Read the model definition and answer for the solid it produces. Units are mm, in the model's axes. Face numbers are marked on the shaded views. Give positions to 0.01 mm unless a question says otherwise; leave off trailing zeros. Order: outer loops, then holes, each group sorted by start corner. A loop starts at its lowest first (then second) coordinate and runs counter-clockwise, first axis right, second up.
```python
from build123d import *

# Parameters (mm, degrees)
F0_W     = 39
F0_H     = 55
F1_DEPTH = 25
F3_DEPTH = 25
F4_R     = 5


with BuildPart() as f1:
    # F0 (on Front) → F1 (new body)
    with BuildSketch(Plane.XZ):
        Rectangle(F0_W, F0_H)
    extrude(amount=F1_DEPTH)

    # F2 (on face) → F3 (cut)
    with BuildSketch(Plane.XZ.offset(25)):
        with BuildLine():
            Line((18.6, 27.5), (-18.6, 27.5))
            ThreePointArc((-18.6, 27.5), (-13.089826, 1.090185), (0, -22.5))
            ThreePointArc((0, -22.5), (13.089826, 1.090185), (18.6, 27.5))
        make_face()
    extrude(amount=-F3_DEPTH, mode=Mode.SUBTRACT)

    # F4
    f4_edges = [f1.edges().sort_by_distance(p)[0] for p in [
        (-19.5, -12.5, -27.5),
        (19.5, -12.5, -27.5),
    ]]
    fillet(f4_edges, radius=F4_R)


solid = f1.part
```
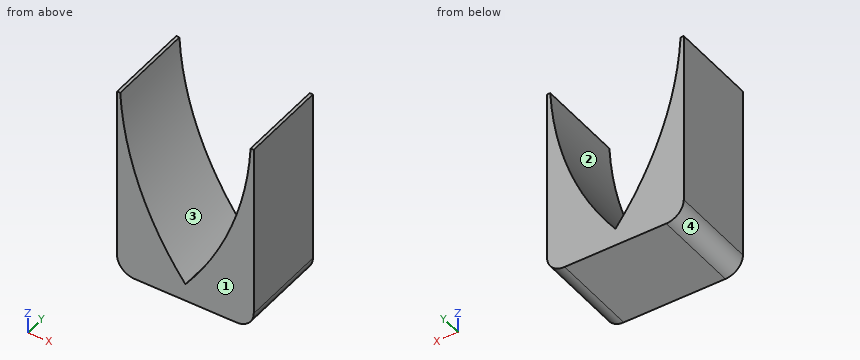
1) The part is cut by section B-B on y = -7.25. Determine the outline of the cut face in (x, z), and give its area (3 significant figures).
Final values:
outline: (-19.5, -22.5) arc R5 ccw to (-14.5, -27.5) - (14.5, -27.5) arc R5 ccw to (19.5, -22.5) - (19.5, 27.5) - (18.6, 27.5) arc R90 cw to (0, -22.5) arc R90 cw to (-18.6, 27.5) - (-19.5, 27.5) - close
area: 915 mm2
2) Consider L1, parallel to X at y = -4.75, z = 20; L2, parallel to X at y = -3.5, z = -10.5; L3, parallel to Z at x = 5, y = -14.5. Determine where each line is inside the solid, lowest interval first.
Final values:
L1: x = -19.5 to -17.87, 17.87 to 19.5
L2: x = -19.5 to -7.82, 7.82 to 19.5
L3: z = -27.5 to -15.32
3) The part is cut by section D-D on x = -12. Determine the outline of the cut face in (y, z).
Final values:
outline: (-25, -27.5) - (0, -27.5) - (0, -1.7) - (-25, -1.7) - close
4) For a pull along X with two mould halves and no side action, classify the marked faces 1, 2, 3 and 4 as released by +X, released by -X, zero draft, split by the parting line, or undercut.
Final values:
face 1: zero draft
face 2: undercut
face 3: undercut
face 4: released by -X
5) The part is cut by section C-C on z = -0.5. Determine the outline of the cut face in (x, y).
Final values:
outline: (-19.5, -25) - (-12.48, -25) - (-12.48, 0) - (-19.5, 0) - close; (12.48, -25) - (19.5, -25) - (19.5, 0) - (12.48, 0) - close
6) The part is cut by section A-A on z = 13. Determine the outline of the cut face in (x, y), and give its area (3 significant figures).
Final values:
outline: (-19.5, -25) - (-16.61, -25) - (-16.61, 0) - (-19.5, 0) - close; (16.61, -25) - (19.5, -25) - (19.5, 0) - (16.61, 0) - close
area: 145 mm2
